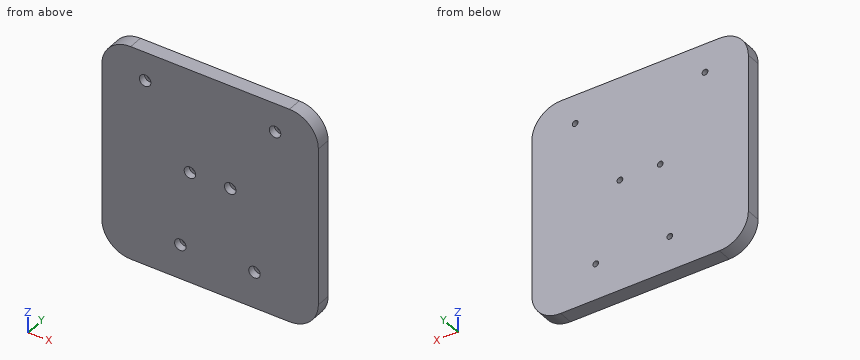
```python
from build123d import *

# Parameters (mm, degrees)
SKETCH1_W           = 150
SKETCH1_H           = 150
SKETCH1_R           = 2
BOSS_EXTRUDE1_DEPTH = 10
SKETCH2_R           = 4
CUT_EXTRUDE1_DEPTH  = 5
FILLET1_R           = 20


with BuildPart() as part:
    # Sketch1 → Boss-Extrude1 (new body)
    with BuildSketch(Plane(origin=(0, 0, 0), x_dir=(1, 0, 0), z_dir=(0, 1, 0))):
        with Locations((75, 75)):
            Rectangle(SKETCH1_W, SKETCH1_H)
        with Locations(Location((30, 20, 0), (0, 0, 270))):
            Circle(SKETCH1_R, mode=Mode.SUBTRACT)
        with Locations(Location((120, 20, 0), (0, 0, 270))):
            Circle(SKETCH1_R, mode=Mode.SUBTRACT)
        with Locations(Location((61.03, 72.42, 0), (0, 0, 270))):
            Circle(SKETCH1_R, mode=Mode.SUBTRACT)
        with Locations(Location((88.97, 72.42, 0), (0, 0, 270))):
            Circle(SKETCH1_R, mode=Mode.SUBTRACT)
        with Locations(Location((105.74, 124.76, 0), (0, 0, 270))):
            Circle(SKETCH1_R, mode=Mode.SUBTRACT)
        with Locations(Location((54.4, 126.03, 0), (0, 0, 270))):
            Circle(SKETCH1_R, mode=Mode.SUBTRACT)
    extrude(amount=BOSS_EXTRUDE1_DEPTH)

    # Sketch2 → Cut-Extrude1 (cut)
    with BuildSketch(Plane.XZ):
        with Locations(Location((30, -20, 0), (0, 0, 270))):
            Circle(SKETCH2_R)
        with Locations(Location((120, -20, 0), (0, 0, 270))):
            Circle(SKETCH2_R)
        with Locations(Location((88.97, -72.42, 0), (0, 0, 270))):
            Circle(SKETCH2_R)
        with Locations(Location((61.03, -72.42, 0), (0, 0, 270))):
            Circle(SKETCH2_R)
        with Locations(Location((54.4, -126.03, 0), (0, 0, 270))):
            Circle(SKETCH2_R)
        with Locations(Location((105.74, -124.76, 0), (0, 0, 270))):
            Circle(SKETCH2_R)
    extrude(amount=-CUT_EXTRUDE1_DEPTH, mode=Mode.SUBTRACT)

    # Fillet1
    fillet1_edges = [part.edges().sort_by_distance(p)[0] for p in [
        (0, 5, -150),
        (150, 5, -150),
        (150, 5, 0),
        (0, 5, 0),
    ]]
    fillet(fillet1_edges, radius=FILLET1_R)


solid = part.part
```
The listing builds one solid part. Answer for the finished solid, in the listing's coordinates (mm). Give positions to 0.01 mm unless a question says otherwise; leave off trailing zeros. Write each loop counter-clockwise with the first axis right and the second up, starting at its lowest first coordinate (ties: lowest second). Pieces come first, ordered by that corner, then holes. Notation, with made-up numbers: (0.5, 5) - (54.5, 5) arc R19 ccw to (54.5, 34) - close; hole circle Ø1 at (47, -7.5). An arc over 180 degrees is marked (long way). Use one line per item in the form item = value. Start each with the question number.
1) Find section C-C on z = -72.5. Determine the outline of the cut face in (x, y), plus the area to 3 significant figures.
2) Find section A-A on y = 1.5. Determine the outline of the cut face in (x, z).
3) Find section B-B on x = 54.4. Determine the outline of the cut face in (y, z), plus the area to 3 significant figures.
4) Flat-ended cylindrical pins translate along their axes: pin 1 Ø4.5 at (x, z) = (88.97, -72.42) entering from -Y; pin 2 Ø1.5 at (y, z) = (3, -135) entering from +X. Find the tip coordinate at first contact, or state that the pin passes through.
5) Consider line 1 along X through (y, z) = (7.35, -72.42); line 2 along Z through (x, y) = (120, 6.15); line 3 along Z through (x, y) = (61, 7.5). Determine where each line is inside the solid, lowest interval first. Write a range as from..to.
Geometry results:
q1.outline = (0, 0) - (57.03, 0) - (57.03, 5) - (59.03, 5) - (59.03, 10) - (0, 10) - close; (63.03, 5) - (65.03, 5) - (65.03, 0) - (84.97, 0) - (84.97, 5) - (86.97, 5) - (86.97, 10) - (63.03, 10) - close; (90.97, 5) - (92.97, 5) - (92.97, 0) - (150, 0) - (150, 10) - (90.97, 10) - close
q1.area = 1,380 mm2
q2.outline = (0, -130) arc R20 ccw to (20, -150) - (130, -150) arc R20 ccw to (150, -130) - (150, -20) arc R20 ccw to (130, 0) - (20, 0) arc R20 ccw to (0, -20) - close; hole circle Ø8 at (30, -20); hole circle Ø8 at (54.4, -126.03); hole circle Ø8 at (61.03, -72.42); hole circle Ø8 at (88.97, -72.42); hole circle Ø8 at (105.74, -124.76); hole circle Ø8 at (120, -20)
q3.outline = (0, -150) - (10, -150) - (10, -128.03) - (5, -128.03) - (5, -130.03) - (0, -130.03) - close; (0, -122.03) - (5, -122.03) - (5, -124.03) - (10, -124.03) - (10, 0) - (0, 0) - close
q3.area = 1,440 mm2
q4.pin_1 = 5
q4.pin_2 = 149.54
q5.line_1 = 0..59.03, 63.03..86.97, 90.97..150
q5.line_2 = -150..-22, -18..0
q5.line_3 = -150..-74.42, -70.42..0
